Part model, mm, in its own coordinate system. Coordinates: 2 decimals unless noted, no trailing zeros. Order: outer loops, then holes, each group sorted by start corner. A loop starts at its lowest first (then second) coordinate and runs counter-clockwise, first axis right, second up.
from build123d import *

# Parameters (mm, degrees)
EXTRUDE_1_DEPTH     = 50
EXTRUDE_2_DEPTH     = 7.5
CUT_EXTRUDE_1_DEPTH = 105.899189701


with BuildPart() as part:
    # 草图1 → 凸台-拉伸1 (new, symmetric)
    with BuildSketch(Plane(origin=(0, 0, 0), x_dir=(1, 0, 0), z_dir=(0, 1, 0))):
        with BuildLine():
            Line((-22, 0), (-20.5, 0))
            ThreePointArc((-20.5, 0), (0, 20.5), (20.5, 0))
            Line((20.5, 0), (22, 0))
            ThreePointArc((22, 0), (15.836666316, 15.270887335), (0.8, 21.985449734))
            ThreePointArc((0.8, 21.985449734), (-15.270887335, 15.836666316), (-22, 0))
        make_face()
    extrude(amount=EXTRUDE_1_DEPTH, both=True)

    # 草图2 → 凸台-拉伸2 (add, symmetric)
    with BuildSketch(Plane(origin=(0, 0, 0), x_dir=(1, 0, 0), z_dir=(0, 1, 0))):
        with BuildLine():
            Line((-0.8, 22.8), (-0.8, 21.985449734))
            ThreePointArc((-0.8, 21.985449734), (0, 22), (0.8, 21.985449734))
            Line((0.8, 21.985449734), (0.8, 22.8))
            Line((0.8, 22.8), (-0.8, 22.8))
        make_face()
    extrude(amount=EXTRUDE_2_DEPTH, both=True)

    # 草图3 → 切除-拉伸1 (cut, through all)
    with BuildSketch(Plane(origin=(0, 50, 0), x_dir=(1, 0, 0), z_dir=(0, 1, 0))):
        Polygon((0, 0), (22, 10.258768479), (22, 0), align=None)
    extrude(amount=-CUT_EXTRUDE_1_DEPTH, mode=Mode.SUBTRACT)


solid = part.part
Q1. Cut at C-C on x = -18. Write the cut outline in (y, z), and give its area (3 significant figures).
Results list:
outline: (-50, -12.65) - (50, -12.65) - (50, -9.81) - (-50, -9.81) - close
area: 284 mm2
Q2. Wall check: line 1 along X through (y, z) = (30, -13.25); line 2 along X through (y, z) = (18, -15.5); line 3 along X through (y, z) = (-22.5, -1.25). Give the ranges that are in metal, low to high.
Results list:
line 1: x = -17.56 to -15.64, 15.64 to 17.56
line 2: x = -15.61 to -13.42, 13.42 to 15.61
line 3: x = -21.96 to -20.46
Q3. Cut at A-A on z = -13.5. Write the cut outline in (x, y).
Results list:
outline: (-17.37, -50) - (-15.43, -50) - (-15.43, 50) - (-17.37, 50) - close; (15.43, -50) - (17.37, -50) - (17.37, 50) - (15.43, 50) - close
Q4. Pin check, flat tips, straight feed: pin 1 Ø12 at (x, y) = (-10, -3.5) entering from +Z; pin 2 Ø0.7 at (x, z) = (0, -22.5) entering from -Y; pin 3 Ø0.9 at (x, z) = (0, -22.5) entering from +Y. Stop position of each tip, or through.
Results list:
pin 1: stops at z = -12.82
pin 2: stops at y = -7.5
pin 3: stops at y = 7.5
Q5. Cut at D-D on y = -3. Write the cut outline in (x, z).
Results list:
outline: (-22, 0) arc R22 ccw to (-0.8, -21.99) - (-0.8, -22.8) - (0.8, -22.8) - (0.8, -21.99) arc R22 ccw to (19.94, -9.3) - (18.58, -8.66) arc R20.5 cw to (-20.5, 0) - close
Q6. Cut at B-B on y = 18.5. Write the cut outline in (x, z), and give its area (3 significant figures).
Results list:
outline: (-22, 0) arc R22 ccw to (19.94, -9.3) - (18.58, -8.66) arc R20.5 cw to (-20.5, 0) - close
area: 86.2 mm2
